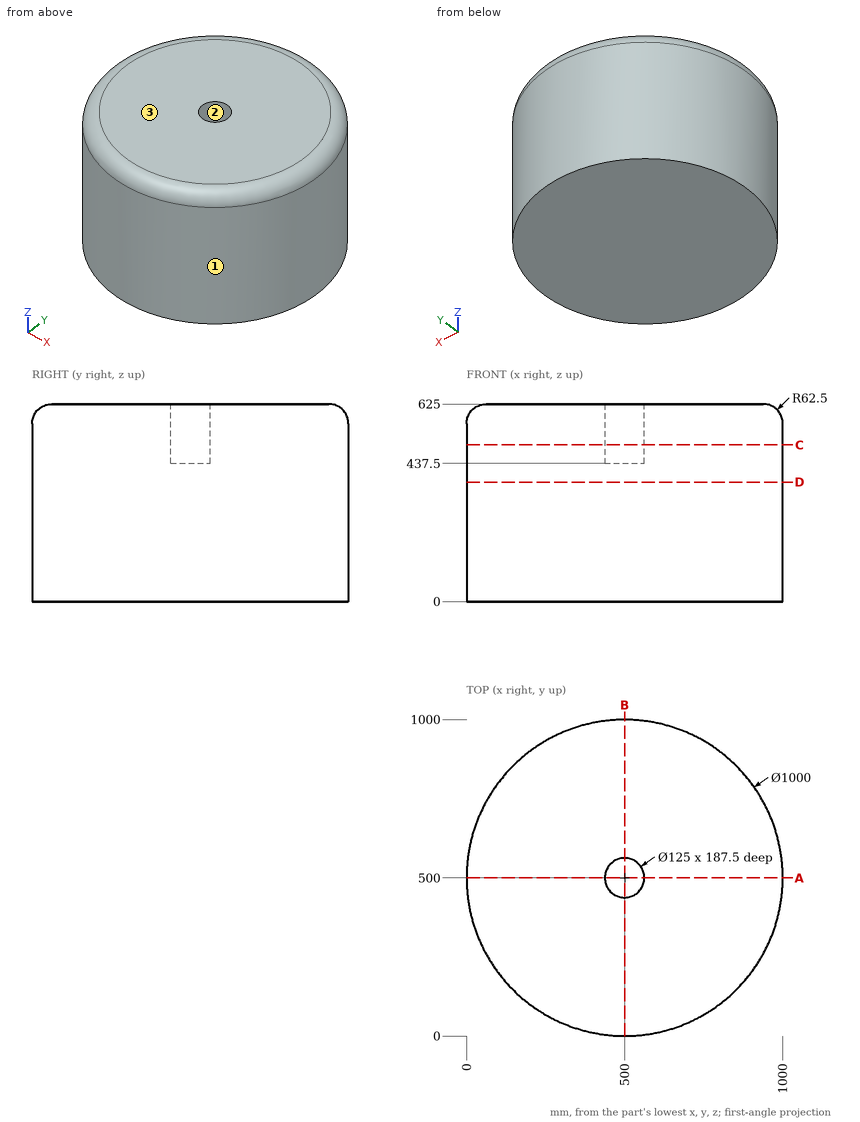
Verification items for this drawing (mm, ordinates from the low corner). Round coordinates to 2 decimals unless told otherwise and drop trailing zeros. Order: outer loops, then holes, each group sorted by start corner. A loop starts at its lowest first (then second) coordinate and runs counter-clockwise, first axis right, second up. Notation, with made-up numbers: (-23.5, 56) -> (15.5, 56) arc R20 cw to (15.5, 65) -> close; hole circle Ø9 at (-31, -16.5). An arc over 180 degrees is marked (long way). Use one line per item in the form item = value.
1. Go/stop test with flat-tipped pins: pin 1 (5 mm diameter, centred on y = 869.5, z = 492.5, fed in from +X); pin 2 (6 mm diameter, centred on y = 180, z = 480, fed in from -X); pin 3 (10 mm diameter, centred on y = 423, z = 534.5, fed in from -X). Record where each tip stops, or that it passes through.
Working result:
pin_1 = 839.57
pin_2 = 113.33
pin_3 = 5.21
2. Cross-section at D-D, the plane z = 378. Enter the section's corners in (x, y).
Working result:
outline = circle Ø1000 at (500, 500)
3. Mould release check, pull along Y, two halves, no side actions. Record for the marked faces 1, 2 and 3: pulls with the +Y half, pulls with the -Y half, needs draft (parallel to the pull), parting line crosses it, or undercut.
Working result:
face_1 = parting line crosses it
face_2 = undercut
face_3 = needs draft
4. Cross-section at A-A, the plane y = 500. Enter the section's corners in (x, z), plus the area to 3 significant figures.
Working result:
outline = (0, 0) -> (1000, 0) -> (1000, 562.5) arc R62.5 ccw to (937.5, 625) -> (562.5, 625) -> (562.5, 437.5) -> (437.5, 437.5) -> (437.5, 625) -> (62.5, 625) arc R62.5 ccw to (0, 562.5) -> close
area = 600,000 mm^2
5. Scan lines: line 1 along Y through (x, z) = (500, 526); line 2 along Y through (x, z) = (663, 121); line 3 along Y through (x, z) = (783, 517). Record each from-to range of solid material in increasing order. Write a range as from..to.
Working result:
line_1 = 0..437.5, 562.5..1000
line_2 = 27.32..972.68
line_3 = 87.8..912.2
6. Cross-section at C-C, the plane z = 495.5. Enter the section's corners in (x, y), plus the area to 3 significant figures.
Working result:
outline = circle Ø1000 at (500, 500); hole circle Ø125 at (500, 500)
area = 773,000 mm^2
